CAD build for the part. Positions are in the model's coordinates, mm. Face numbers are marked on the shaded views. A direction names the side the tool comes from. Give positions to 0.01 mm unless a question says otherwise; leave off trailing zeros. Loops run counter-clockwise (first coordinate to the right, second up) from the corner with the lowest first, then second, coordinate; pieces in that order, holes last.
```python
from build123d import *

# Parameters (mm, degrees)
PAD_DEPTH    = 2
SKETCH001_W  = 2
SKETCH001_H  = 34.122
PAD001_DEPTH = 32.6


with BuildPart() as part:
    # Sketch → Pad (new body)
    with BuildSketch(Plane.YZ):
        Polygon((-23.355, 0), (23.355, 0), (23.355, 13.665881), (-31.245, 13.665881), align=None)
    extrude(amount=PAD_DEPTH)

    # Sketch001 (on Face6 of Pad) → Pad001 (join)
    with BuildSketch(Plane.YZ.offset(2)):
        with Locations((0, 17.061)):
            Rectangle(SKETCH001_W, SKETCH001_H)
    extrude(amount=PAD001_DEPTH)


solid = part.part
```
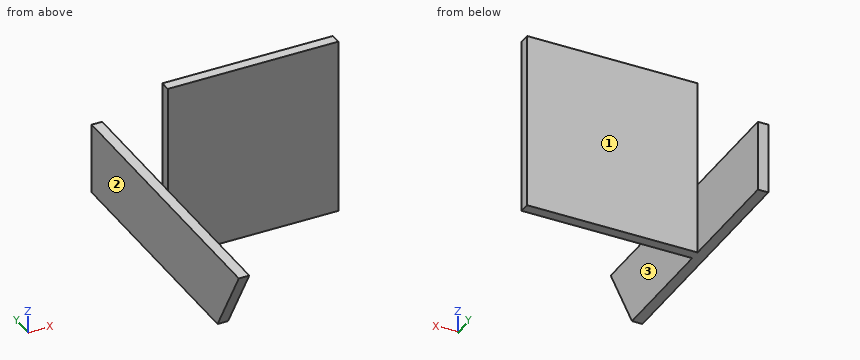
1. Saw through at D-D, the plane z = 5.5. List the corners of the cut face in (x, y) (3 decimals), and give its area (3 significant figures).
Responses:
outline: (0, -26.53) - (2, -26.53) - (2, -1) - (34.6, -1) - (34.6, 1) - (2, 1) - (2, 23.355) - (0, 23.355) - close
area: 165 mm2
2. Tool access for the marked faces 1, 2 and 3: list every direction of +Z, -Z, +X, -X, +Y, -Y with a clear straight run to the whole face (end or side of a thin tool).
Responses:
face 1: +Z, -Z, +X, +Y
face 2: +Z, -Z, -X, +Y, -Y
face 3: +Z, -Z, +X, -Y
3. Saw through at C-C, the plane y = -22. List the corners of the cut face in (x, z).
Responses:
outline: (0, 0) - (2, 0) - (2, 13.67) - (0, 13.67) - close
4. Saw through at A-A, the plane z = 10. List the corners of the cut face in (x, y) (1 decimal), and give its area (3 significant figures).
Responses:
outline: (0, -29.1) - (2, -29.1) - (2, -1) - (34.6, -1) - (34.6, 1) - (2, 1) - (2, 23.4) - (0, 23.4) - close
area: 170 mm2
5. Saw through at B-B, the plane x = 26.5. List the corners of the cut face in (y, z).
Responses:
outline: (-1, 0) - (1, 0) - (1, 34.12) - (-1, 34.12) - close
6. Drop flat-ended pins along their axis: pin 1 (2 mm diameter, centred on y = 0, z = 21.5, fed in from -X); pin 2 (7 mm diameter, centred on y = 17, z = 3.5, fed in from +X); pin 3 (4 mm diameter, centred on y = -10.5, z = 9.5, fed in from -X); pin 4 (3 mm diameter, centred on x = 15.5, z = 18.5, fed in from +Y). Give the stop position or say it passes through.
Responses:
pin 1: stops at x = 2
pin 2: stops at x = 2
pin 3: stops at x = 0
pin 4: stops at y = 1
7. Probe line 1 along Y through (x, z) = (21, 24.5); line 2 along X through (y, z) = (-6.5, 3); line 3 along X through (y, z) = (0, 17.5). List the from-to ranges inside material, lowest first.
Responses:
line 1: y = -1 to 1
line 2: x = 0 to 2
line 3: x = 2 to 34.6
